Drawing for the job (mm, zero at the part's lowest x, y, z). A direction names the side the tool comes from. Coordinates: 2 decimals unless noted, no trailing zeros. Write each loop counter-clockwise with the first axis right and the second up, starting at its lowest first coordinate (ties: lowest second). Pieces come first, ordered by that corner, then holes. Notation, with made-up numbers: (-9.5, 66.25) - (22.5, 66.25) arc R22 ccw to (22.5, 105.25) - close; hole circle Ø2 at (-10, -29). An arc over 180 degrees is marked (long way). Write each question's results on one line, items separated by ' | '.
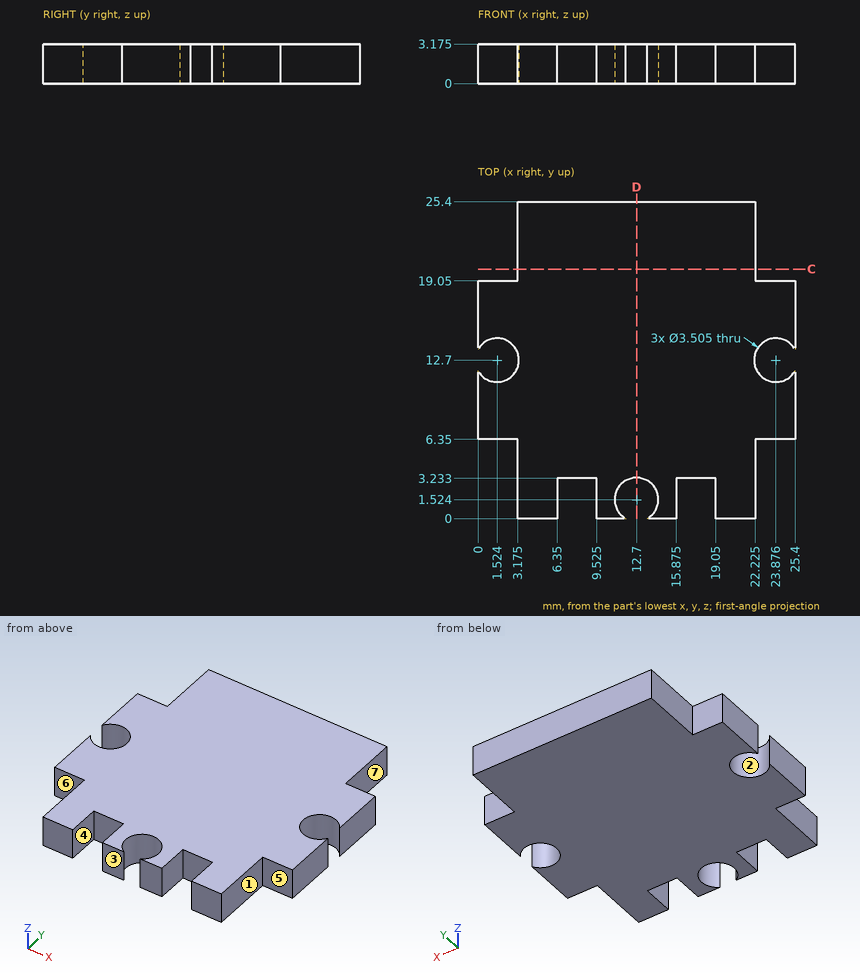
(1) Two-plate mould, pull along X, no slides. Class the marked faces 1, 2 and 3: released by +X, released by -X, zero draft, split by the parting line, or undercut.
Return value:
face 1: released by +X | face 2: undercut | face 3: zero draft
(2) Saw through at C-C on y = 20. Write the cut outline in (x, z) (3 decimals).
Return value:
outline: (3.175, 0) - (22.225, 0) - (22.225, 3.175) - (3.175, 3.175) - close
(3) Saw through at D-D on x = 12.7. Write the cut outline in (y, z) (1 decimal).
Return value:
outline: (3.3, 0) - (25.4, 0) - (25.4, 3.2) - (3.3, 3.2) - close
(4) Wall check: line 1 (Y direction, x = 1.5, z = 2.6); line 2 (Y direction, x = 6.5, z = 2.95); line 3 (Y direction, x = 12.7, z = 0.6). Give the ranges that are in metal, low to high. Write a range as from..to.
Return value:
line 1: y = 6.35..10.95, 14.45..19.05 | line 2: y = 3.23..25.4 | line 3: y = 3.28..25.4
(5) Flat gauge pins, fed straight in: P1, Ø1, axis at y = 1.5, z = 1.5, coming from the +X side (3 decimals); P2, Ø1, axis at y = 21.5, z = 1.5, coming from the -X side (3 decimals). Where does each tip first touch, or does it go through?
Return value:
P1: stops at x = 22.225 | P2: stops at x = 3.175
(6) 3-axis set-ups, long thin cutter, end or side, ignore diameter. For the marked faces 4, 5, 6 and 7: which of +Z, -Z, +X, -X, +Y, -Y reach the whole face in a straight line?
Return value:
face 4: +Z, -Z, -Y | face 5: +Z, -Z, +X, -Y | face 6: +Z, -Z, -X, -Y | face 7: +Z, -Z, +X, +Y
